Check sheet for the modelled part. Datum: model origin and axes. Units: mm. A direction names the side the tool comes from. Round coordinates to 2 decimals unless told otherwise and drop trailing zeros. Order: outer loops, then holes, each group sorted by start corner. A loop starts at its lowest first (then second) coordinate and runs counter-clockwise, first axis right, second up. Notation, with made-up numbers: (75.5, -31.5) -> (88.5, -31.5) arc R23 ccw to (88.5, -18.5) -> close; hole circle Ø11 at (-9, 4). An arc over 180 degrees is marked (long way). Answer in a Markdown table with one row per item. Add a question column.
1. Material ranges on L1, parallel to Y at x = 0, z = 1; L2, parallel to Z at x = -0.15, y = 38.5; L3, parallel to Z at x = -24, y = 15, recorded low to high. Write a range as from..to.
2. Access from +Z, -Z, +X, -X, +Y, -Y to the whole of each face (thin tool, end or side, straight path). Record for faces 5 (the flat face through (0.65, 36, 1)), 6 (the flat face through (-5, 33, 1)), 7 (the flat face through (10, 33, 1)).
3. Depth check by flat-ended pin: P1, Ø2, axis at x = 2.5, z = 1, coming from the +Y side; P2, Ø1, axis at x = 20.5, z = 1, coming from the +Y side; P3, Ø2, axis at y = 38.5, z = 1, coming from the -X side. Enter the tip coordinate at first touch or a pass-through.
4. Sectioned sample at D-D, the plane x = -23.5. Record the boundary of the cut face in (y, z).
5. Draft check along Y on faces 1 (the flat face through (-3, 32.5, 1)), 2 (the flat face through (-10, 33, 1)), 3 (the flat face through (5, 33, 1)), 4 (the cylindrical face through (-28.986, -26.797, 0.986)). Enter one of: +Y half, -Y half, draft (parallel to the pull), parting line (faces both ways), or undercut.
6. Sectioned sample at B-B, the plane x = -7. Record the boundary of the cut face in (y, z), then the cut area to 3 significant figures.
7. Sectioned sample at A-A, the plane x = 12.5. Record the boundary of the cut face in (y, z), then the cut area to 3 significant figures.
8. Sectioned sample at C-C, the plane y = -9.5. Record the boundary of the cut face in (x, z).
```python
from build123d import *

# Parameters (mm, degrees)
BOSS_EXTRUDE1_DEPTH = 2
BOSS_EXTRUDE2_DEPTH = 30
CUT_EXTRUDE2_DEPTH  = 25
SKETCH4_R           = 0.8
BOSS_EXTRUDE3_DEPTH = 0.65


with BuildPart() as part:
    # Sketch2 → Boss-Extrude1 (new body)
    with BuildSketch(Plane.XY):
        with BuildLine():
            Line((15, -32.5), (-15, -32.5))
            ThreePointArc((-15, -32.5), (-29.142135624, -26.642135624), (-35, -12.5))
            Line((-35, -12.5), (-35, 32.5))
            Line((-35, 32.5), (35, 32.5))
            Line((35, 32.5), (35, -12.5))
            ThreePointArc((35, -12.5), (29.142135624, -26.642135624), (15, -32.5))
        make_face()
    extrude(amount=BOSS_EXTRUDE1_DEPTH)

    # Sketch3 → Boss-Extrude2 (add)
    with BuildSketch(Plane(origin=(35, 0, 0), x_dir=(0, 0, -1), z_dir=(1, 0, 0))):
        with BuildLine():
            Line((-2, 32.5), (-1, 32.5))
            Line((-1, 32.5), (-1, 34.5))
            ThreePointArc((-1, 34.5), (-2.931851653, 33.01763809), (-2, 30.767949192))
            Line((-2, 30.767949192), (-2, 32.5))
        make_face()
        with BuildLine():
            Line((-1, 34.5), (-1, 32.5))
            Line((-1, 32.5), (0, 32.5))
            Line((0, 32.5), (0, 30.767949192))
            ThreePointArc((0, 30.767949192), (0.732050808, 31.5), (1, 32.5))
            ThreePointArc((1, 32.5), (0.414213562, 33.914213562), (-1, 34.5))
        make_face()
        with BuildLine():
            Line((0, 32.5), (-1, 32.5))
            Line((-1, 32.5), (-2, 32.5))
            Line((-2, 32.5), (-2, 30.767949192))
            ThreePointArc((-2, 30.767949192), (-1, 30.5), (0, 30.767949192))
            Line((0, 30.767949192), (0, 32.5))
        make_face()
        with BuildLine():
            ThreePointArc((-2, 30.767949192), (-2.931851653, 33.01763809), (-1, 34.5))
            Line((-1, 34.5), (-1, 35))
            ThreePointArc((-1, 35), (-3.447265782, 33.010774109), (-2, 30.208712153))
            Line((-2, 30.208712153), (-2, 30.767949192))
        make_face()
        with BuildLine():
            Line((-1, 35), (-1, 34.5))
            ThreePointArc((-1, 34.5), (0.414213562, 33.914213562), (1, 32.5))
            ThreePointArc((1, 32.5), (0.732050808, 31.5), (0, 30.767949192))
            Line((0, 30.767949192), (0, 30.208712153))
            ThreePointArc((0, 30.208712153), (1.091650066, 31.130693606), (1.5, 32.5))
            ThreePointArc((1.5, 32.5), (0.767766953, 34.267766953), (-1, 35))
        make_face()
        with BuildLine():
            ThreePointArc((0, 30.767949192), (-1, 30.5), (-2, 30.767949192))
            Line((-2, 30.767949192), (-2, 30.208712153))
            ThreePointArc((-2, 30.208712153), (-1, 30), (0, 30.208712153))
            Line((0, 30.208712153), (0, 30.767949192))
        make_face()
    boss_extrude2 = extrude(amount=-BOSS_EXTRUDE2_DEPTH)

    # Sketch3_4 → Cut-Extrude2 (cut)
    with BuildSketch(Plane(origin=(35, 0, 0), x_dir=(0, 0, -1), z_dir=(1, 0, 0))):
        with BuildLine():
            Line((-2, 32.5), (-1, 32.5))
            Line((-1, 32.5), (-1, 34.5))
            ThreePointArc((-1, 34.5), (-2.931851653, 33.01763809), (-2, 30.767949192))
            Line((-2, 30.767949192), (-2, 32.5))
        make_face()
        with BuildLine():
            Line((0, 32.5), (-1, 32.5))
            Line((-1, 32.5), (-2, 32.5))
            Line((-2, 32.5), (-2, 30.767949192))
            ThreePointArc((-2, 30.767949192), (-1, 30.5), (0, 30.767949192))
            Line((0, 30.767949192), (0, 32.5))
        make_face()
        with BuildLine():
            Line((-1, 34.5), (-1, 32.5))
            Line((-1, 32.5), (0, 32.5))
            Line((0, 32.5), (0, 30.767949192))
            ThreePointArc((0, 30.767949192), (0.732050808, 31.5), (1, 32.5))
            ThreePointArc((1, 32.5), (0.414213562, 33.914213562), (-1, 34.5))
        make_face()
    cut_extrude2 = extrude(amount=-CUT_EXTRUDE2_DEPTH, mode=Mode.SUBTRACT)

    # Mirror1: Boss-Extrude2, Cut-Extrude2 across plane
    add(boss_extrude2.mirror(Plane(origin=(0, 0, 0), x_dir=(0, 0, 1), z_dir=(1, 0, 0))))
    add(cut_extrude2.mirror(Plane(origin=(0, 0, 0), x_dir=(0, 0, 1), z_dir=(1, 0, 0))), mode=Mode.SUBTRACT)

    # Sketch4 → Boss-Extrude3 (add, symmetric)
    with BuildSketch(Plane(origin=(0, 0, 0), x_dir=(0, 0, -1), z_dir=(1, 0, 0))):
        with BuildLine():
            Line((-2, 37.063859338), (-2, 32.5))
            Line((-2, 32.5), (0, 32.5))
            Line((0, 32.5), (0, 37.063859338))
            ThreePointArc((0, 37.063859338), (-1, 40.25), (-2, 37.063859338))
        make_face()
        with Locations((-1, 38.5)):
            Circle(SKETCH4_R, mode=Mode.SUBTRACT)
    extrude(amount=BOSS_EXTRUDE3_DEPTH, both=True)


solid = part.part
```
Answer key:
| question | item | result |
|---|---|---|
| 1 | L1 | y = -32.5..37.7, 39.3..40.25 |
| 1 | L2 | z = -0.75..0.2, 1.8..2.75 |
| 1 | L3 | z = 0..2 |
| 2 | face 5 | +Z, -Z, +Y |
| 2 | face 6 | +Y |
| 2 | face 7 | +X |
| 3 | P1 | stops at y = 32.5 |
| 3 | P2 | stops at y = 35 |
| 3 | P3 | stops at x = -0.65 |
| 4 | outline | (-30.6, 0) -> (30.21, 0) arc R2.5 ccw (long way) to (30.21, 2) -> (-30.6, 2) -> close; hole circle Ø4 at (32.5, 1) |
| 5 | face 1 | +Y half |
| 5 | face 2 | undercut |
| 5 | face 3 | draft |
| 5 | face 4 | -Y half |
| 6 | outline | (-32.5, 0) -> (30.21, 0) arc R2.5 ccw (long way) to (30.21, 2) -> (-32.5, 2) -> close |
| 6 | area | 145 mm² |
| 7 | outline | (-32.5, 0) -> (30.21, 0) arc R2.5 ccw (long way) to (30.21, 2) -> (-32.5, 2) -> close; hole circle Ø4 at (32.5, 1) |
| 7 | area | 132 mm² |
| 8 | outline | (-35, 0) -> (35, 0) -> (35, 2) -> (-35, 2) -> close |
